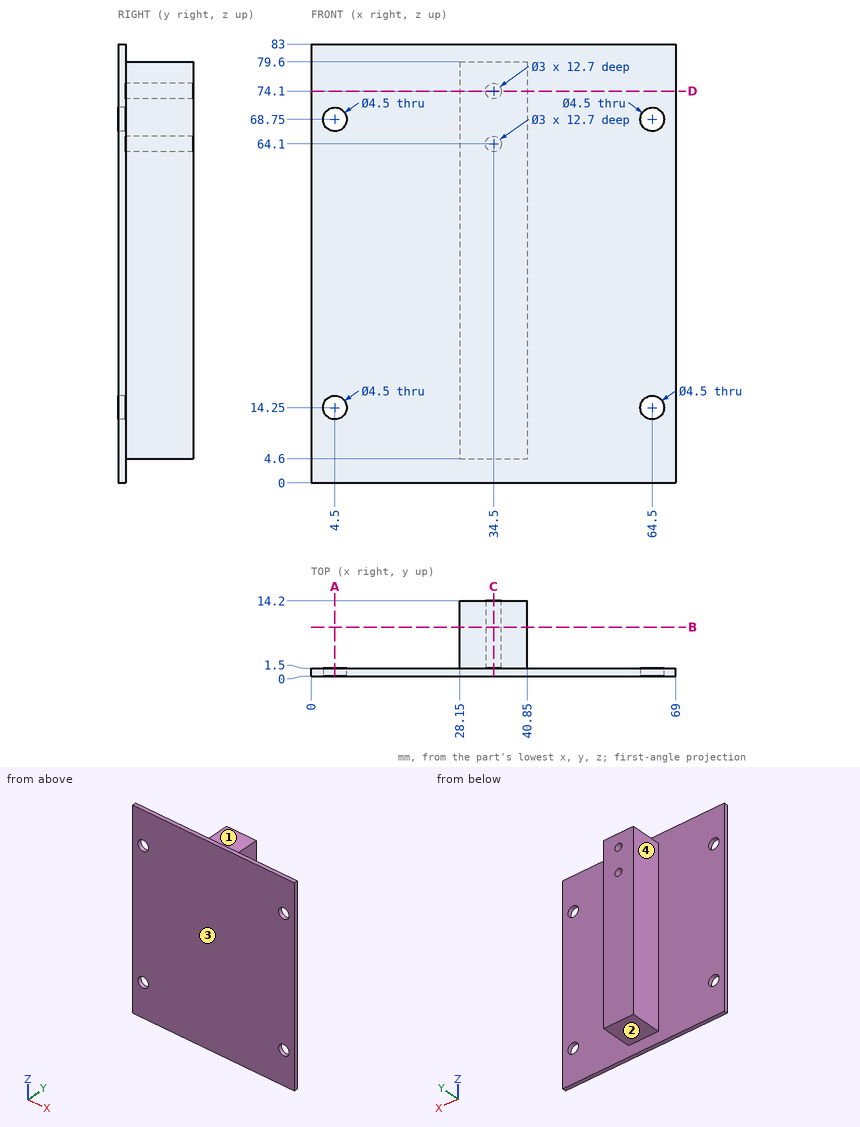
Design review of the part shown in the three views and the two pictorial views. Dimensions are in mm from the part's minimum x, y and z. A direction names the side the tool comes from. Give positions to 0.01 mm unless a question says otherwise; leave off trailing zeros. Write each loop counter-clockwise with the first axis right and the second up, starting at its lowest first coordinate (ties: lowest second). Pieces come first, ordered by that corner, then holes.
Item 1: Take a section at C-C (x = 34.5). Give the boundary of the cut face in (y, z), and give its area (3 significant figures).
Item 2: Machinability: for the marked faces 1, 2, 3 and 4, which of the approach directions +Z, -Z, +X, -X, +Y, -Y give a long, thin tool a straight path to every point of the face, cutting with its end or side? Answer none if there is none.
Item 3: Wall thickness on probe 1 along Z at (x, y) = (4.5, 0.8); probe 2 along X at (y, z) = (0.6, 14.25); probe 3 along Z at (x, y) = (34.5, 9.75): over which ranges is each line inside the solid? List them lowest first.
Item 4: Take a section at D-D (z = 74.1). Give the boundary of the cut face in (x, y), and give its area (3 significant figures).
Item 5: Insertion check: P1, Ø1, axis at y = 2.5, z = 34.5, coming from the -X side; P2, Ø3.5, axis at x = 4.5, z = 14.25, coming from the +Y side; P3, Ø6.5, axis at x = 36.5, y = 11, coming from the -Z side; P4, Ø5, axis at y = 5.5, z = 40, coming from the +X side. Each pin has a flat end and moves straight along its axis. Give the tip position at first contact, or say it passes through.
Item 6: Take a section at A-A (x = 4.5). Give the boundary of the cut face in (y, z), and give its area (3 significant figures).
Item 7: Take a section at B-B (y = 9.25). Give the boundary of the cut face in (x, z), and give its area (3 significant figures).
Established:
1. outline: (0, 0) - (1.5, 0) - (1.5, 4.6) - (14.2, 4.6) - (14.2, 62.6) - (1.5, 62.6) - (1.5, 65.6) - (14.2, 65.6) - (14.2, 72.6) - (1.5, 72.6) - (1.5, 75.6) - (14.2, 75.6) - (14.2, 79.6) - (1.5, 79.6) - (1.5, 83) - (0, 83) - close
1. area: 1,000 mm2
2. face 1: +Z, +X, -X, +Y
2. face 2: -Z, +X, -X, +Y
2. face 3: +Z, -Z, +X, -X, -Y
2. face 4: +Z, -Z, -X, +Y
3. probe 1: z = 0 to 12, 16.5 to 66.5, 71 to 83
3. probe 2: x = 0 to 2.25, 6.75 to 62.25, 66.75 to 69
3. probe 3: z = 4.6 to 62.6, 65.6 to 72.6, 75.6 to 79.6
4. outline: (0, 0) - (69, 0) - (69, 1.5) - (40.85, 1.5) - (40.85, 14.2) - (36, 14.2) - (36, 1.5) - (33, 1.5) - (33, 14.2) - (28.15, 14.2) - (28.15, 1.5) - (0, 1.5) - close
4. area: 227 mm2
5. P1: stops at x = 28.15
5. P2: passes through
5. P3: stops at z = 4.6
5. P4: stops at x = 40.85
6. outline: (0, 0) - (1.5, 0) - (1.5, 12) - (0, 12) - close; (0, 16.5) - (1.5, 16.5) - (1.5, 66.5) - (0, 66.5) - close; (0, 71) - (1.5, 71) - (1.5, 83) - (0, 83) - close
6. area: 111 mm2
7. outline: (28.15, 4.6) - (40.85, 4.6) - (40.85, 79.6) - (28.15, 79.6) - close; hole circle Ø3 at (34.5, 64.1); hole circle Ø3 at (34.5, 74.1)
7. area: 938 mm2
